Could you check a few things on this model? Use its own coordinates, in mm. Give positions to 0.01 mm unless a question says otherwise; leave off trailing zeros. Loops run counter-clockwise (first coordinate to the right, second up) from the corner with the lowest first, then second, coordinate; pieces in that order, holes last. Notation, with made-up numbers: M -18.75,-4 L 26.25,-4 A17 ccw 26.25,9 Z; hole C 71.5,8 d1. An arc over 180 degrees is marked long. Use CSV: the item, a comma, the result in double quotes.
```python
from build123d import *

# Parameters (mm, degrees)
BOSS_EXTRUDE1_DEPTH = 81
SKETCH2_OUTSIDE_W   = 22.24
SKETCH2_OUTSIDE_H   = 22.24
SKETCH2_OUTSIDE_R   = 2
CUT_EXTRUDE3_DEPTH  = 82
FILLET1_R           = 0.5


with BuildPart() as part:
    # Sketch1 → Boss-Extrude1 (new body)
    with BuildSketch(Plane.XY):
        Polygon((-1, 1), (-1, 2), (1, 2), (1, 1), (2, 1), (2, -1), (1, -1), (1, -2), (-1, -2), (-1, -1), (-2, -1), (-2, 1), align=None)
    extrude(amount=BOSS_EXTRUDE1_DEPTH)

    # Sketch2 outside → Cut-Extrude3 (cut, through all)
    with BuildSketch(Plane.XY):
        Rectangle(SKETCH2_OUTSIDE_W, SKETCH2_OUTSIDE_H)
        Circle(SKETCH2_OUTSIDE_R, mode=Mode.SUBTRACT)
    extrude(amount=CUT_EXTRUDE3_DEPTH, mode=Mode.SUBTRACT)

    # Fillet1
    fillet1_edges = [part.edges().sort_by_distance(p)[0] for p in [
        (1.366025404, -1, 0),
        (-1, -1.366025404, 0),
        (-1.366025404, 1, 0),
        (1, 1.366025404, 0),
        (-1.366025404, 1, 81),
        (-1, -1.366025404, 81),
        (1.366025404, 1, 0),
        (1, -1.366025404, 0),
        (-1.366025404, -1, 0),
        (-1, 1.366025404, 0),
        (-2, 0, 0),
        (0, 2, 0),
        (2, 0, 0),
        (0, -2, 0),
        (1.366025404, -1, 81),
        (-1, 1.366025404, 81),
        (-1.366025404, -1, 81),
        (1, -1.366025404, 81),
        (1.366025404, 1, 81),
        (1, 1.366025404, 81),
        (0, 2, 81),
        (-2, 0, 81),
        (0, -2, 81),
        (2, 0, 81),
    ]]
    fillet(fillet1_edges, radius=FILLET1_R)


solid = part.part
```
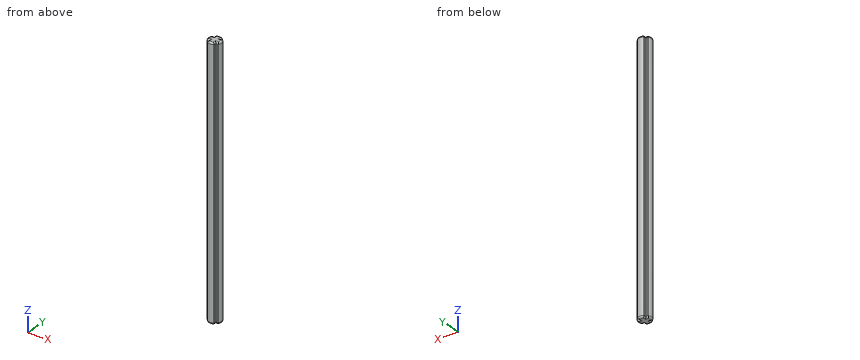
1. Please list where these lines run through material, in increasing order: line 1 (Y direction, x = -1.05, z = 22); line 2 (Y direction, x = 0.15, z = 77.5).
Outcome:
line 1,"-1 to 1"
line 2,"-1.99 to 1.99"
2. I'm going to push flat-ended pins straight in: pin 1 Ø2 at (y, z) = (1.5, 62.5) entering from +X; pin 2 Ø0.8 at (x, z) = (-1.5, 43) entering from -Y; pin 3 Ø0.6 at (x, z) = (1.5, 54) entering from +Y. Where does each tip first touch, or does it pass through?
Outcome:
pin 1,"x = 1.94"
pin 2,"y = -1"
pin 3,"y = 1"
3. I want a section at A-A, the plane z = 37. List the corners of the cut face in (x, y) for me, then the cut area to 3 significant figures.
Outcome:
outline,"M -1.73,-1 L -1,-1 L -1,-1.73 A2 ccw 1,-1.73 L 1,-1 L 1.73,-1 A2 ccw 1.73,1 L 1,1 L 1,1.73 A2 ccw -1,1.73 L -1,1 L -1.73,1 A2 ccw Z"
area,"11.3 mm2"
